The model under review builds one solid part; all positions refer to its coordinate system, in mm. A direction names the side the tool comes from. Round coordinates to 2 decimals unless told otherwise and drop trailing zeros. Order: outer loops, then holes, each group sorted by start corner. A loop starts at its lowest first (then second) coordinate and runs counter-clockwise, first axis right, second up.
1) Consider section B-B (z = -0.7). Give the boundary of the cut face in (x, y), then the cut area to 3 significant figures.
2) Mouldability with a two-part tool opening along X and no side actions: class faces 1 (the face through (-2.5, 4, 0)), 2 (the face through (1.5, 4, 0)), 3 (the face through (2, 7.5, 0)) as pulls with the +X half, pulls with the -X half, needs draft (parallel to the pull), parting line crosses it, or undercut.
3) To check wall thickness, follow L1, parallel to X at y = 4.75, z = 2.15; L2, parallel to X at y = 2.5, z = 1.05; L3, parallel to Y at x = 0.8, z = -0.35. State the ranges of each line that lie inside material, in increasing order.
4) Clearance check with a flat-ended pin moving along its axis: P1, Ø1.5, axis at x = 0.5, z = -0.5, coming from the +Y side. State where the tip first meets the part, or that it passes through.
5) Consider section C-C (x = 0). Give the boundary of the cut face in (y, z), then the cut area to 3 significant figures.
6) Consider section A-A (y = 4.25). Give the boundary of the cut face in (x, z).
7) Machinability: for faces 4 (the face through (-1, 5, 2)), 5 (the face through (-1.5, 4, 0)), 6 (the face through (2.5, 4, 0)), which of the approach directions +Z, -Z, +X, -X, +Y, -Y give a long, thin tool a straight path to every point of the face, cutting with its end or side? Answer none if there is none.
Autodesk Inventor part; units mm, degrees
ref_plane "YZ Plane" through (0, 0, 0) normal (1, 0, 0) x (0, 1, 0)
ref_plane "XZ Plane" through (0, 0, 0) normal (0, 1, 0) x (-1, 0, 0)
ref_plane "XY Plane" through (0, 0, 0) normal (0, 0, 1) x (1, 0, 0)
sketch "Sketch1" plane through (0, 0, 0) normal (0, 1, 0) x (-1, 0, 0)
  line L0 (-2.5, 2.5) -> (2.5, 2.5)
  line L1 (2.5, 2.5) -> (2.5, -2.5)
  line L2 (2.5, -2.5) -> (-2.5, -2.5)
  line L3 (-2.5, -2.5) -> (-2.5, 2.5)
  line L4 (-2.5, 2.5) -> (2.5, -2.5) construction
  line L5 (2.5, 2.5) -> (-2.5, -2.5) construction
  point P0 (0, 0)
  dimension "d0" = 5
  dimension "d1" = 5
extrude "Extrusion1" add sketch "Sketch1" along normal blind 7.5
shell "Shell1" thickness 1 removed faces 1 at (-0.8333, 7.5, -0.8333)
sketch "Sketch3" plane through (-2.5, 0, 2.5) normal (0, 0, 1) x (1, 0, 0)
  line L0 (2.5, 9.1674) -> (2.5, 2.1156) construction
  line L1 (1.4995, 9.1674) -> (1.4995, 2.1156)
  line L2 (3.5005, 2.1156) -> (3.5005, 9.1674)
  arc A0 (3.5005, 9.1674) -> (1.4995, 9.1674) centre (2.5, 9.1674) ccw
  arc A1 (1.4995, 2.1156) -> (3.5005, 2.1156) centre (2.5, 2.1156) ccw
  point P0 (2.5, 0)
  point P1 (2.5, 5.6415)
extrude "Extrusion3" cut sketch "Sketch3" against normal through all
properties part number "snapfit_v04"
Answer below:
1. outline: (-2.5, 0) - (2.5, 0) - (2.5, 7.5) - (1.5, 7.5) - (1.5, 1) - (-1.5, 1) - (-1.5, 7.5) - (-2.5, 7.5) - close
1. area: 18.0 mm2
2. face 1: pulls with the -X half
2. face 2: undercut
2. face 3: needs draft
3. L1: x = -2.5 to -1, 1 to 2.5
3. L2: x = -2.5 to -1.5, 1.5 to 2.5
3. L3: y = 0 to 1
4. P1: stops at y = 1
5. outline: (0, -2.5) - (1.12, -2.5) - (1.12, -1.5) - (1, -1.5) - (1, 1.5) - (1.12, 1.5) - (1.12, 2.5) - (0, 2.5) - close
5. area: 5.23 mm2
6. outline: (-2.5, -2.5) - (-1, -2.5) - (-1, -1.5) - (-1.5, -1.5) - (-1.5, 1.5) - (-1, 1.5) - (-1, 2.5) - (-2.5, 2.5) - close; (1, -2.5) - (2.5, -2.5) - (2.5, 2.5) - (1, 2.5) - (1, 1.5) - (1.5, 1.5) - (1.5, -1.5) - (1, -1.5) - close
7. face 4: +Z, -Z, +Y
7. face 5: +Y
7. face 6: +Z, -Z, +X, +Y, -Y
